Geometry: final body of the model. Coordinates: model frame, mm. A direction names the side the tool comes from. Give positions to 0.01 mm unless a question says otherwise; leave off trailing zeros. Order: outer loops, then holes, each group sorted by start corner. A loop starts at its lowest first (then second) coordinate and runs counter-clockwise, first axis right, second up. Notation, with made-up numbers: (26, 26.25) - (70, 26.25) arc R27 cw to (70, 65.25) - close; hole circle Ø9 at (69.25, 14). An arc over 180 degrees is marked (long way). One line per item, written item: value.
```python
from build123d import *

# Parameters (mm, degrees)
F0_W     = 60
F0_H     = 50
F1_DEPTH = 5
F2_W     = 5
F2_H     = 25
F3_DEPTH = 30
F4_R     = 12.49999
F5_R     = 2.5
F6_DEPTH = 50


# Not quite as in the source:
# - a fillet or chamfer is up to 0.001 mm smaller than in the source, because OpenCascade refuses the exact size


with BuildPart() as f1:
    # F0 (on Top) → F1 (new body)
    with BuildSketch(Plane.XY):
        Rectangle(F0_W, F0_H)
    extrude(amount=F1_DEPTH)

    # F2 (on face) → F3 (join)
    with BuildSketch(Plane.XY.offset(5)):
        with Locations((-11.5, 0)):
            Rectangle(F2_W, F2_H)
        with Locations((11.5, 0)):
            Rectangle(F2_W, F2_H)
    extrude(amount=F3_DEPTH)

    # F4 (radius 12.5 in the source; OpenCascade refuses exactly that, so slightly less here)
    f4_edges = [f1.edges().sort_by_distance(p)[0] for p in [
        (-11.5, -12.5, 35),
        (-11.5, 12.5, 35),
        (11.5, 12.5, 35),
        (11.5, -12.5, 35),
    ]]
    fillet(f4_edges, radius=F4_R)

    # F5 (on face) → F6 (cut)
    with BuildSketch(Plane(origin=(-14, 0, 0), x_dir=(0, -1, 0), z_dir=(-1, 0, 0))):
        with Locations((0, 22.5)):
            Circle(F5_R)
    extrude(amount=-F6_DEPTH, mode=Mode.SUBTRACT)


solid = f1.part
```
1) Mould query, pull axis Y, two halves, no side actions, for faces 5 (the face through (11.535, -8.935, 31.241)), 6 (the face through (11, 0, 25)), 7 (the face through (14, -0.2, 19.8)). Classes: released by +Y, released by -Y, zero draft, split by the parting line, or undercut.
Answers below:
face 5: released by -Y
face 6: undercut
face 7: zero draft
2) Section D-D, the plane z = 29. Return loops of the section in (x, y), then the cut area to 3 significant figures.
Answers below:
outline: (-14, -10.68) - (-9, -10.68) - (-9, 10.68) - (-14, 10.68) - close; (9, -10.68) - (14, -10.68) - (14, 10.68) - (9, 10.68) - close
area: 214 mm^2
3) Section A-A, the plane z = 10. Return loops of the section in (x, y).
Answers below:
outline: (-14, -12.5) - (-9, -12.5) - (-9, 12.5) - (-14, 12.5) - close; (9, -12.5) - (14, -12.5) - (14, 12.5) - (9, 12.5) - close
4) Section B-B, the plane x = -7.5. Return loops of the section in (y, z), then the cut area to 3 significant figures.
Answers below:
outline: (-25, 0) - (25, 0) - (25, 5) - (-25, 5) - close
area: 250 mm^2
5) Material intervals for line 1 along X through (y, z) = (8, 6); line 2 along Z through (x, y) = (12, 0); line 3 along Z through (x, y) = (11.5, -15.5), sorted ascending.
Answers below:
line 1: -14 to -9, 9 to 14
line 2: 0 to 20, 25 to 35
line 3: 0 to 5
6) Section C-C, the plane y = -11.5. Return loops of the section in (x, z), then the cut area to 3 significant figures.
Answers below:
outline: (-30, 0) - (30, 0) - (30, 5) - (14, 5) - (14, 27.4) - (9, 27.4) - (9, 5) - (-9, 5) - (-9, 27.4) - (-14, 27.4) - (-14, 5) - (-30, 5) - close
area: 524 mm^2
7) Set-up query: faces 1 (the face through (-12, 12.5, 14)), 2 (the face through (-12, -12.5, 14)), 3 (the face through (-14, -0.2, 19.8)), 4 (the face through (9, -0.2, 19.8)). Return all of +Z, -Z, +X, -X, +Y, -Y with unobstructed straight access to the full face (end or side cutting, diameter ignored); none if empty.
Answers below:
face 1: +Z, +X, -X, +Y
face 2: +Z, +X, -X, -Y
face 3: +Z, -X, +Y, -Y
face 4: +Z, +Y, -Y
8) First-contact query: pin 1 (3 mm diameter, centred on y = 0, z = 22.5, fed in from -X) (3 decimals); pin 2 (4 mm diameter, centred on y = -3.5, z = 25, fed in from -X); pin 3 (12.5 mm diameter, centred on y = 5.5, z = 16.5, fed in from +X); pin 4 (1.5 mm diameter, centred on x = 12.5, z = 11, fed in from -Y). Flat tips, straight axial feed; report the tip coordinate or a pass-through.
Answers below:
pin 1: through
pin 2: x = -14
pin 3: x = 14
pin 4: y = -12.5
